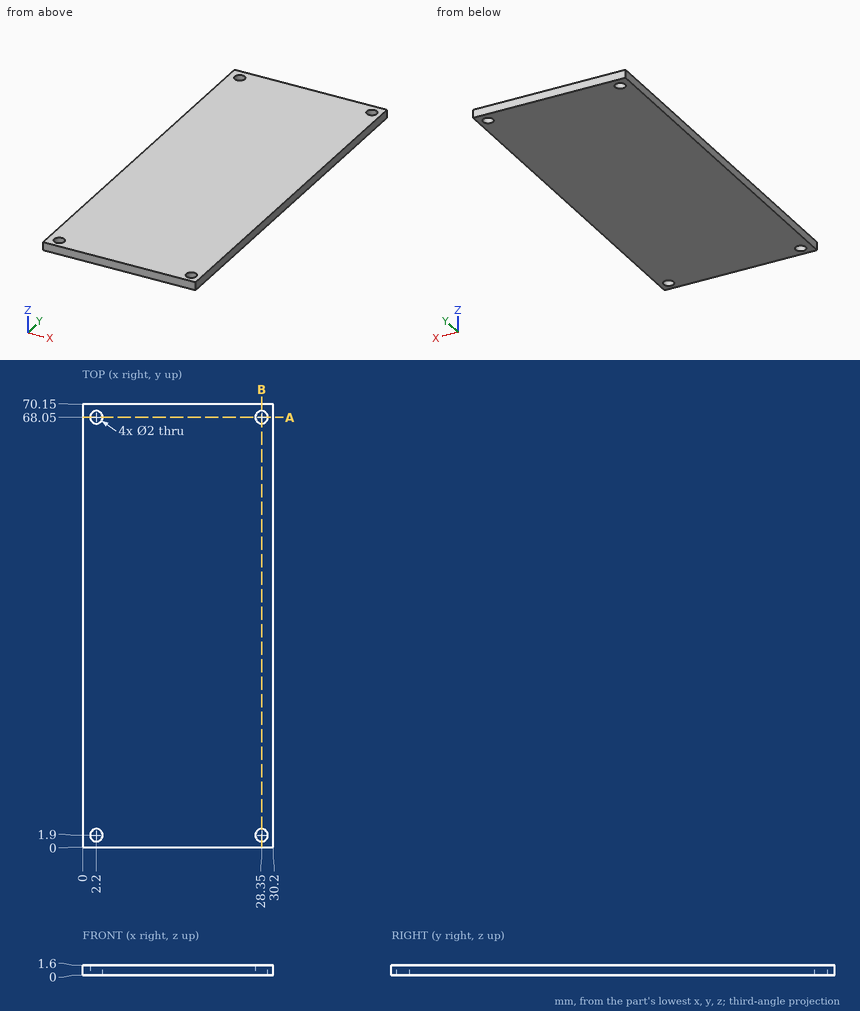
Source: three-view drawing plus pictorial views. Frame: mm from the lowest corner of the part. Give positions to 0.01 mm unless a question says otherwise; leave off trailing zeros. Loops run counter-clockwise (first coordinate to the right, second up) from the corner with the lowest first, then second, coordinate; pieces in that order, holes last.
1) Section query B-B on x = 28.35. Return the cut outline in (y, z), and give its area (3 significant figures).
A:
outline: (0, 0) - (0.9, 0) - (0.9, 1.6) - (0, 1.6) - close; (2.9, 0) - (67.05, 0) - (67.05, 1.6) - (2.9, 1.6) - close; (69.05, 0) - (70.15, 0) - (70.15, 1.6) - (69.05, 1.6) - close
area: 106 mm2
2) Section query A-A on y = 68.05. Return the cut outline in (x, z).
A:
outline: (0, 0) - (1.2, 0) - (1.2, 1.6) - (0, 1.6) - close; (3.2, 0) - (27.35, 0) - (27.35, 1.6) - (3.2, 1.6) - close; (29.35, 0) - (30.2, 0) - (30.2, 1.6) - (29.35, 1.6) - close
3) Line query: L1, parallel to X at y = 68.05, z = 1; L2, parallel to Y at x = 2.2, z = 1.35. Output: solid intervals per line, ascending.
A:
L1: x = 0 to 1.2, 3.2 to 27.35, 29.35 to 30.2
L2: y = 0 to 0.9, 2.9 to 67.05, 69.05 to 70.15
